from build123d import *

# Parameters (mm, degrees)
SKETCH1_W           = 78.5
SKETCH1_H           = 37.4
BOSS_EXTRUDE1_DEPTH = 9.5
SKETCH6_R           = 2
CUT_EXTRUDE1_DEPTH  = 6.5
BOSS_EXTRUDE2_DEPTH = 4
SKETCH9_W           = 13
SKETCH9_H           = 5.5
CUT_EXTRUDE3_DEPTH  = 56.75233179
BOSS_EXTRUDE3_REACH = 83.737
BOSS_EXTRUDE4_START = -4
BOSS_EXTRUDE4_DEPTH = 4
BOSS_EXTRUDE5_DEPTH = 4


with BuildPart() as part:
    # Sketch1 → Boss-Extrude1 (new body)
    with BuildSketch(Plane(origin=(0, 0, 0), x_dir=(1, 0, 0), z_dir=(0, 1, 0))):
        Rectangle(SKETCH1_W, SKETCH1_H)
    extrude(amount=BOSS_EXTRUDE1_DEPTH)

    # Sketch6 → Cut-Extrude1 (cut)
    with BuildSketch(Plane(origin=(0, 9.5, 0), x_dir=(1, 0, 0), z_dir=(0, 1, 0))):
        with Locations(Location((-34.25, 13.7, 0), (0, 0, 270))):
            Circle(SKETCH6_R)
        with Locations(Location((0, 13.7, 0), (0, 0, 270))):
            Circle(SKETCH6_R)
        with Locations(Location((34.25, 13.7, 0), (0, 0, 270))):
            Circle(SKETCH6_R)
        with Locations(Location((34.25, -13.7, 0), (0, 0, 270))):
            Circle(SKETCH6_R)
        with Locations(Location((0, -13.7, 0), (0, 0, 270))):
            Circle(SKETCH6_R)
        with Locations(Location((-34.25, -13.7, 0), (0, 0, 270))):
            Circle(SKETCH6_R)
    extrude(amount=-CUT_EXTRUDE1_DEPTH, mode=Mode.SUBTRACT)

    # Sketch7 → Boss-Extrude2 (add)
    with BuildSketch(Plane.ZY.offset(39.25)):
        with BuildLine():
            Line((-18.7, 0), (-9.037433155, -9.344774046))
            ThreePointArc((-9.037433155, -9.344774046), (0, -13), (9.037433155, -9.344774046))
            Line((9.037433155, -9.344774046), (18.7, 0))
            Line((18.7, 0), (-18.7, 0))
        make_face()
    boss_extrude2 = extrude(amount=-BOSS_EXTRUDE2_DEPTH)

    # Mirror1: Boss-Extrude2 across plane
    add(boss_extrude2.mirror(Plane(origin=(0, 0, 0), x_dir=(0, 0, 1), z_dir=(1, 0, 0))))

    # Sketch9 → Cut-Extrude3 (cut, through all)
    with BuildSketch(Plane(origin=(0, 0, -18.7), x_dir=(-1, 0, 0), z_dir=(0, 0, -1))):
        with Locations((22.75, 4.75)):
            Rectangle(SKETCH9_W, SKETCH9_H)
        with Locations((-22.75, 4.75)):
            Rectangle(SKETCH9_W, SKETCH9_H)
    extrude(amount=-CUT_EXTRUDE3_DEPTH, mode=Mode.SUBTRACT)

    # Boss-Extrude3: up to this face of the body (flat: up to its plane)
    boss_extrude3_end = Plane(part.part.faces().sort_by_distance((-39.25, 0.189608499, 0))[0])
    # Sketch10 → Boss-Extrude3 (add, up to the picked face)
    with BuildSketch(Plane(origin=(39.25, 0, 0), x_dir=(0, 0, -1), z_dir=(1, 0, 0)), mode=Mode.PRIVATE) as boss_extrude3_sk1:
        with BuildLine():
            Line((-22.7, -40.5), (-24.7, -40.5))
            Line((-24.7, -40.5), (-24.7, 9.5))
            Line((-24.7, 9.5), (-18.7, 9.5))
            Line((-18.7, 9.5), (-18.7, 7.5))
            ThreePointArc((-18.7, 7.5), (-21.528427125, 6.328427125), (-22.7, 3.5))
            Line((-22.7, 3.5), (-22.7, -40.5))
        make_face()
    boss_extrude3_tool1 = split(extrude(boss_extrude3_sk1.sketch, amount=-BOSS_EXTRUDE3_REACH, mode=Mode.PRIVATE), bisect_by=boss_extrude3_end, keep=Keep.BOTH, mode=Mode.PRIVATE)
    add(boss_extrude3_tool1.solids().sort_by(Axis((39.25, -13.095828, 23.426281), (-1, 0, 0)))[0])

    # Sketch11 → Boss-Extrude4 (add)
    with BuildSketch(Plane.ZY.offset(39.25).offset(BOSS_EXTRUDE4_START)):
        with BuildLine():
            Line((18.7, 7.5), (18.7, 0))
            ThreePointArc((18.7, 0), (21.261557408, 0.476218058), (22.7, -1.696163792))
            Line((22.7, -1.696163792), (22.7, 3.5))
            ThreePointArc((22.7, 3.5), (21.528427125, 6.328427125), (18.7, 7.5))
        make_face()
    extrude(amount=BOSS_EXTRUDE4_DEPTH)

    # Sketch12 → Boss-Extrude5 (add)
    with BuildSketch(Plane(origin=(39.25, 0, 0), x_dir=(0, 0, -1), z_dir=(1, 0, 0))):
        with BuildLine():
            Line((-18.7, 0), (-18.7, 7.5))
            ThreePointArc((-18.7, 7.5), (-21.528427125, 6.328427125), (-22.7, 3.5))
            Line((-22.7, 3.5), (-22.7, -1.696163792))
            ThreePointArc((-22.7, -1.696163792), (-21.261557408, 0.476218058), (-18.7, 0))
        make_face()
    extrude(amount=-BOSS_EXTRUDE5_DEPTH)


solid = part.part
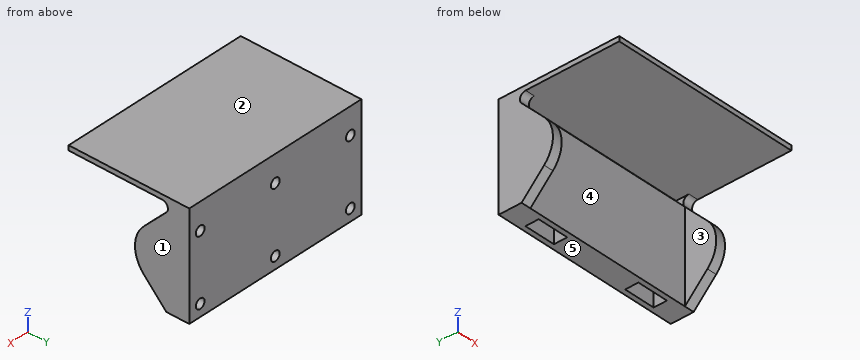
The model under review builds one solid part; all positions refer to its coordinate system, in mm. Face numbers are marked on the shaded views. A direction names the side the tool comes from. Round coordinates to 2 decimals unless told otherwise and drop trailing zeros. Loops run counter-clockwise (first coordinate to the right, second up) from the corner with the lowest first, then second, coordinate; pieces in that order, holes last. Notation, with made-up numbers: M 13.25,66.25 L 68.25,66.25 A28 cw 68.25,104.25 Z; hole C 38,48 d10. An arc over 180 degrees is marked long. Answer as CSV lines item,"result".
1. We need section B-B (y = -5). Give the boundary of the cut face in (x, z), plus the area to 3 significant figures.
Outcome:
outline,"M -39.25,-13.53 L -35.25,-13.53 L -35.25,13.53 L -39.25,13.53 Z; M -39.25,22.7 L 39.25,22.7 L 39.25,24.7 L -39.25,24.7 Z; M 35.25,-13.53 L 39.25,-13.53 L 39.25,13.53 L 35.25,13.53 Z"
area,"373 mm2"
2. We need section C-C (z = -13.7). Give the boundary of the cut face in (x, y).
Outcome:
outline,"M -39.25,-4.84 L -35.25,-4.84 L -35.25,0 L 35.25,0 L 35.25,-4.84 L 39.25,-4.84 L 39.25,9.5 L 36.25,9.5 L 36.25,3 L 32.25,3 L 32.25,9.5 L 2,9.5 L 2,3 L -2,3 L -2,9.5 L -32.25,9.5 L -32.25,3 L -36.25,3 L -36.25,9.5 L -39.25,9.5 Z; hole M -29.25,2 L -16.25,2 L -16.25,7.5 L -29.25,7.5 Z; hole M 16.25,2 L 29.25,2 L 29.25,7.5 L 16.25,7.5 Z"
3. Draft analysis for pull direction X (two halves, no side actions). For the marked faces 1, 2 and 3, state which applies: pulls with the +X half, pulls with the -X half, needs draft (parallel to the pull), parting line crosses it, or undercut.
Outcome:
face 1,"pulls with the +X half"
face 2,"needs draft"
face 3,"undercut"
4. For the marked faces 4 and 5, list the 3-axis set-ups (+Z, -Z, +X, -X, +Y, -Y) from which the entire face can be reached by the end or side of a thin tool; tool diameter is ignored.
Outcome:
face 4,"-Z, -Y"
face 5,"-Z, +X, -X, +Y, -Y"
5. To check wall thickness, follow L1, parallel to Y at x = 20.5, z = -7; L2, parallel to X at y = 5, z = -13; L3, parallel to Z at x = 34, y = 5. State the ranges of each line that lie inside material, in increasing order. Write a range as [from, to].
Outcome:
L1,"y = [0, 2], [7.5, 9.5]"
L2,"x = [-39.25, -36.12], [-32.38, -29.25], [-16.25, -1.87], [1.87, 16.25], [29.25, 32.38], [36.12, 39.25]"
L3,"z = [-18.7, -15.68], [-11.72, 11.72], [15.68, 18.7], [22.41, 24.7]"
6. We need section A-A (x = -21). Give the boundary of the cut face in (y, z).
Outcome:
outline,"M -40.5,22.7 L 3.5,22.7 A4 cw 7.5,18.7 L 7.5,-18.7 L 9.5,-18.7 L 9.5,24.7 L -40.5,24.7 Z; M 0,-18.7 L 2,-18.7 L 2,18.7 L 0,18.7 Z"
7. Insertion check: pin 1 Ø2 at (x, z) = (-34, 14.5) entering from +Y; pin 2 Ø3 at (x, z) = (-1, 13) entering from +Y; pin 3 Ø2 at (x, y) = (8, -18) entering from -Z; pin 4 Ø6 at (x, z) = (-24, -12.5) entering from -Y. Each pin has a flat end and moves straight along its axis. Give the tip position at first contact, or say it passes through.
Outcome:
pin 1,"stops at y = 3"
pin 2,"stops at y = 9.5"
pin 3,"stops at z = 22.7"
pin 4,"stops at y = 0"
8. We need section D-D (x = 0). Give the boundary of the cut face in (y, z).
Outcome:
outline,"M -40.5,22.7 L 3.5,22.7 A4 cw 7.5,18.7 L 0,18.7 L 0,-18.7 L 9.5,-18.7 L 9.5,-15.7 L 3,-15.7 L 3,-11.7 L 9.5,-11.7 L 9.5,11.7 L 3,11.7 L 3,15.7 L 9.5,15.7 L 9.5,24.7 L -40.5,24.7 Z"
